Can you work these out from the drawing? Everything is in mm from the part's minimum corner. A direction names the side the tool comes from. Give positions to 0.01 mm unless a question says otherwise; leave off trailing zeros. Write each loop counter-clockwise with the first axis right and the second up, starting at its lowest first coordinate (ties: lowest second). Pieces come first, ordered by that corner, then holes. Notation, with made-up numbers: M 8.5,26.5 L 38.5,26.5 A6 cw 38.5,32.5 Z; hole C 69.25,-16.75 d7. An arc over 180 degrees is marked long. One line per item, written item: value.
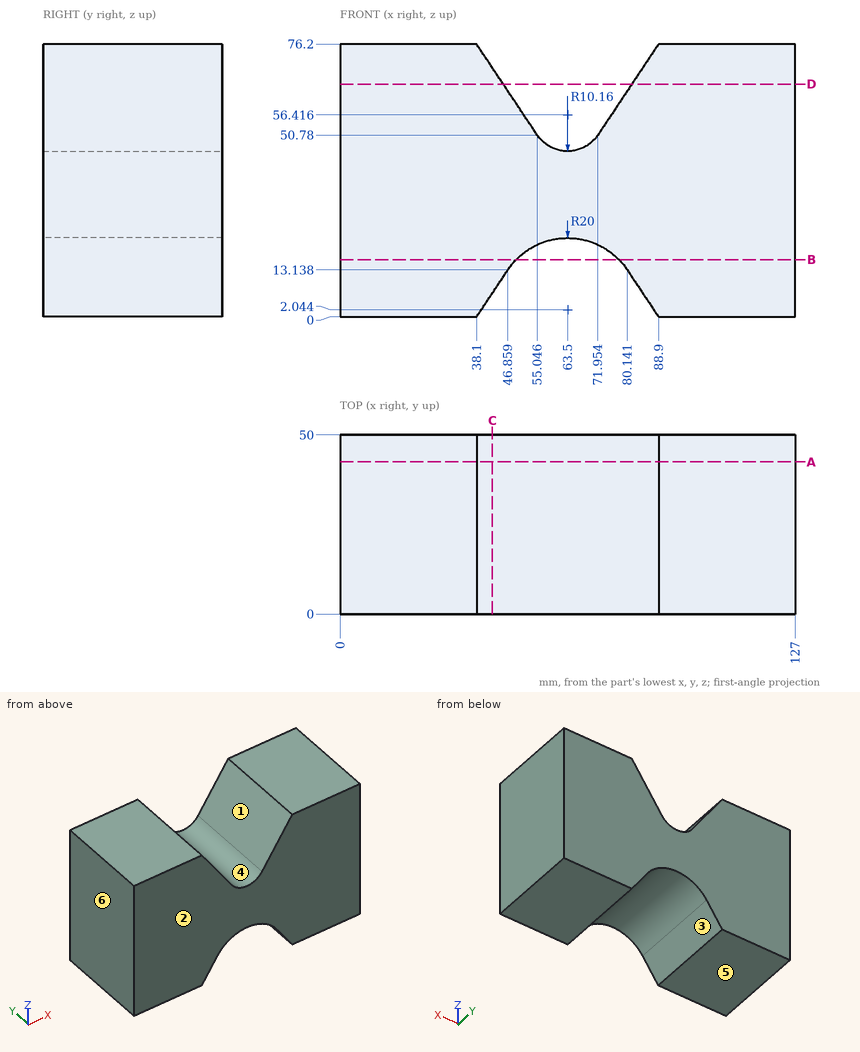
1) On a 3-axis mill with a long thin cutter (end or side, diameter ignored), from which of +Z, -Z, +X, -X, +Y, -Y can I reach the whole of each face in a straight line? I mean the marked faces 1, 2 and 3. Say none if no direction works.
Outcome:
face 1: +Z, +Y, -Y
face 2: +Z, -Z, +X, -X, -Y
face 3: -Z, +Y, -Y
2) If we section it at B-B, the plane z = 16: Write out the boundary of the cut face in (x, y), then the cut area to 3 significant figures.
Outcome:
outline: M 0,0 L 49.17,0 L 49.17,50 L 0,50 Z; M 77.83,0 L 127,0 L 127,50 L 77.83,50 Z
area: 4,920 mm^2
3) If we section it at C-C, the plane x = 42.5: Write out the boundary of the cut face in (y, z).
Outcome:
outline: M 0,6.6 L 50,6.6 L 50,69.6 L 0,69.6 Z
4) Please list where these lines run through material, in increasing order: L1, parallel to X at y = 35, z = 9.5 (1 decimal); L2, parallel to X at y = 8, z = 4.5; L3, parallel to Z at x = 68, y = 7.5. Write a range as from..to.
Outcome:
L1: x = 0..44.4, 82.6..127
L2: x = 0..41.1, 85.9..127
L3: z = 21.53..47.31
5) If we section it at A-A, the plane y = 42.5: Write out the boundary of the cut face in (x, z) (1 decimal).
Outcome:
outline: M 0,0 L 38.1,0 L 46.9,13.1 A20 cw 80.1,13.1 L 88.9,0 L 127,0 L 127,76.2 L 88.9,76.2 L 72,50.8 A10.2 cw 55,50.8 L 38.1,76.2 L 0,76.2 Z
6) I'm going to push flat-ended pins straight in: pin 1 (1.5 mm diameter, centred on x = 48, y = 12.5, fed in from +Z) (1 decimal); pin 2 (2 mm diameter, centred on x = 50.5, y = 11.5, fed in from +Z); pin 3 (4 mm diameter, centred on x = 48, y = 20, fed in from -Z). Where does each tip first touch, or does it pass through?
Outcome:
pin 1: stops at z = 62.5
pin 2: stops at z = 59.1
pin 3: stops at z = 11.85
7) We'd pull the mould along X, two halves only. Please class the marked faces 4, 5 and 6: pulls with the +X half, pulls with the -X half, needs draft (parallel to the pull), parting line crosses it, or undercut.
Outcome:
face 4: undercut
face 5: needs draft
face 6: pulls with the -X half
8) If we section it at D-D, the plane z = 65: Write out the boundary of the cut face in (x, y), then the cut area to 3 significant figures.
Outcome:
outline: M 0,0 L 45.57,0 L 45.57,50 L 0,50 Z; M 81.43,0 L 127,0 L 127,50 L 81.43,50 Z
area: 4,560 mm^2
